```python
from build123d import *

# Parameters (mm, degrees)
SKETCH1_W               = 300
SKETCH1_H               = 300
SKETCH1_W_2             = 180
SKETCH1_H_2             = 200
BOSS_EXTRUDE1_DEPTH     = 8
CUT_EXTRUDE1_DEPTH      = 213.282830205
SKETCH3_R               = 1.5
CUT_EXTRUDE2_DEPTH      = 16.5
SKETCH4_R               = 6
CUT_EXTRUDE4_DEPTH      = 213.282830205
MIRROR4_COPY_1_DEPTH    = 213.282830205
MIRROR4_COPY_2_SKETCH_R = 1.5
MIRROR4_COPY_2_DEPTH    = 16.5
SKETCH5_W               = 200
SKETCH5_H               = 4
CUT_EXTRUDE5_DEPTH      = 213.282830205


with BuildPart() as part:
    # Sketch1 → Boss-Extrude1 (new body)
    with BuildSketch(Plane(origin=(0, 0, 0), x_dir=(1, 0, 0), z_dir=(0, 1, 0))):
        Rectangle(SKETCH1_W, SKETCH1_H)
        with Locations((-10, 0)):
            Rectangle(SKETCH1_W_2, SKETCH1_H_2, mode=Mode.SUBTRACT)
    extrude(amount=BOSS_EXTRUDE1_DEPTH)

    # Sketch2 → Cut-Extrude1 (cut, through all)
    with BuildSketch(Plane(origin=(0, 0, 0), x_dir=(1, 0, 0), z_dir=(0, 1, 0))):
        with BuildLine():
            Line((133.5, 150), (134.5, 150))
            Line((134.5, 150), (134.5, 139.979130372))
            ThreePointArc((134.5, 139.979130372), (134, 128), (133.5, 139.979130372))
            Line((133.5, 139.979130372), (133.5, 150))
        make_face()
    cut_extrude1 = extrude(amount=CUT_EXTRUDE1_DEPTH, mode=Mode.SUBTRACT)

    # Sketch3 → Cut-Extrude2 (cut)
    with BuildSketch(Plane(origin=(150, 0, 0), x_dir=(0, 0, -1), z_dir=(1, 0, 0))):
        with Locations((147.5, 4)):
            Circle(SKETCH3_R)
    cut_extrude2 = extrude(amount=-CUT_EXTRUDE2_DEPTH, mode=Mode.SUBTRACT)

    # Mirror3: Cut-Extrude1, Cut-Extrude2 across plane
    add(cut_extrude1.mirror(Plane.XY), mode=Mode.SUBTRACT)
    add(cut_extrude2.mirror(Plane.XY), mode=Mode.SUBTRACT)

    # Sketch4 → Cut-Extrude4 (cut, through all)
    with BuildSketch(Plane(origin=(0, 0, 0), x_dir=(1, 0, 0), z_dir=(0, 1, 0))):
        with Locations(Location((126, 0, 0), (0, 0, 270))):
            Circle(SKETCH4_R)
    extrude(amount=CUT_EXTRUDE4_DEPTH, mode=Mode.SUBTRACT)

    # Mirror4: Cut-Extrude1, Cut-Extrude2 across plane
    add(cut_extrude1.mirror(Plane(origin=(0, 0, 0), x_dir=(0, 0, 1), z_dir=(1, 0, 0))), mode=Mode.SUBTRACT)
    add(cut_extrude2.mirror(Plane(origin=(0, 0, 0), x_dir=(0, 0, 1), z_dir=(1, 0, 0))), mode=Mode.SUBTRACT)

    # Mirror4 copy 1 sketch → Mirror4 copy 1 (cut, through all)
    with BuildSketch(Plane(origin=(0, 0, 0), x_dir=(-1, 0, 0), z_dir=(0, 1, 0))):
        with BuildLine():
            Line((133.5, 150), (134.5, 150))
            Line((134.5, 150), (134.5, 139.979130372))
            ThreePointArc((134.5, 139.979130372), (134, 128), (133.5, 139.979130372))
            Line((133.5, 139.979130372), (133.5, 150))
        make_face()
    extrude(amount=MIRROR4_COPY_1_DEPTH, mode=Mode.SUBTRACT)

    # Mirror4 copy 2 sketch → Mirror4 copy 2 (cut)
    with BuildSketch(Plane.ZY.offset(150)):
        with Locations((147.5, 4)):
            Circle(MIRROR4_COPY_2_SKETCH_R)
    extrude(amount=-MIRROR4_COPY_2_DEPTH, mode=Mode.SUBTRACT)

    # Sketch5 → Cut-Extrude5 (cut, through all)
    with BuildSketch(Plane(origin=(0, 0, 0), x_dir=(1, 0, 0), z_dir=(0, 1, 0))):
        with Locations((0, 134)):
            Rectangle(SKETCH5_W, SKETCH5_H)
    cut_extrude5 = extrude(amount=CUT_EXTRUDE5_DEPTH, mode=Mode.SUBTRACT)

    # Mirror5: Cut-Extrude5 across plane
    add(cut_extrude5.mirror(Plane.XY), mode=Mode.SUBTRACT)


solid = part.part
```
Source: CAD feature listing. Evaluate the final solid. Frame: model axes, mm. A direction names the side the tool comes from. Give positions to 0.01 mm unless a question says otherwise; leave off trailing zeros. Loops run counter-clockwise (first coordinate to the right, second up) from the corner with the lowest first, then second, coordinate; pieces in that order, holes last. Notation, with made-up numbers: (55.5, 26) -> (82.5, 26) arc R29 cw to (82.5, 51) -> close; hole circle Ø1 at (-22, -31). An arc over 180 degrees is marked (long way). Put each result on its own line as item: value. Start each with the question number.
1) Draft query along Z for faces 1 (the face through (-102, 8, -2)), 2 (the face through (-1, 4, 132)), 3 (the face through (-142, 4, 150)). Return one class per face: released by +Z, released by -Z, zero draft, split by the parting line, or undercut.
2) Material intervals for probe 1 along Z at (x, y) = (68, 4); probe 2 along X at (y, z) = (3.5, 0); probe 3 along X at (y, z) = (4.75, -134), sorted ascending.
3) Cut plane C-C (z = 0). Return loops of the section in (x, y), then the cut area to 3 significant figures.
4) Cut plane B-B (x = 60). Return loops of the section in (y, z), then the cut area to 3 significant figures.
5) Cut plane A-A (z = -56.5). Return loops of the section in (x, y).
6) Reachability of faces 4 (the face through (142, 4, 150)), 5 (the face through (133.5, 4, -145)), 6 (the face through (133.5, 4, 145)), 7 (the face through (-100, 4, 1)), 8 (the face through (-142, 4, -150)) from +Z, -Z, +X, -X, +Y, -Y: full face, straight path, thin tool, end or side. Return the list, or none.
Results are:
1. face 1: zero draft
1. face 2: undercut
1. face 3: released by +Z
2. probe 1: z = -150 to -136, -132 to -100, 100 to 132, 136 to 150
2. probe 2: x = -150 to -100, 80 to 120, 132 to 150
2. probe 3: x = -150 to -140, -128 to -100, 100 to 128, 140 to 150
3. outline: (-150, 0) -> (-100, 0) -> (-100, 8) -> (-150, 8) -> close; (80, 0) -> (120, 0) -> (120, 8) -> (80, 8) -> close; (132, 0) -> (150, 0) -> (150, 8) -> (132, 8) -> close
3. area: 864 mm2
4. outline: (0, -150) -> (8, -150) -> (8, -136) -> (0, -136) -> close; (0, -132) -> (8, -132) -> (8, -100) -> (0, -100) -> close; (0, 100) -> (8, 100) -> (8, 132) -> (0, 132) -> close; (0, 136) -> (8, 136) -> (8, 150) -> (0, 150) -> close
4. area: 736 mm2
5. outline: (-150, 0) -> (-100, 0) -> (-100, 8) -> (-150, 8) -> close; (80, 0) -> (150, 0) -> (150, 8) -> (80, 8) -> close
6. face 4: +Z, +X, -X, +Y, -Y
6. face 5: -Z, +Y, -Y
6. face 6: +Z, +Y, -Y
6. face 7: +Y, -Y
6. face 8: -Z, +X, -X, +Y, -Y
